Autodesk Inventor part; units mm, degrees
ref_plane "YZ Plane" through (0, 0, 0) normal (1, 0, 0) x (0, 1, 0)
ref_plane "XZ Plane" through (0, 0, 0) normal (0, 1, 0) x (-1, 0, 0)
ref_plane "XY Plane" through (0, 0, 0) normal (0, 0, 1) x (1, 0, 0)
sketch "Sketch2" plane through (0, 0, 0) normal (0, 0, 1) x (1, 0, 0)
  circle A0 centre (-22.5, 0) radius 1.2295
  circle A1 centre (11.25, -19.4856) radius 1.2295
  circle A2 centre (11.25, 19.4856) radius 1.2295
  circle A3 centre (22.5, 0) radius 1.2295
  circle A4 centre (-11.25, -19.4856) radius 1.2295
  circle A5 centre (-11.25, 19.4856) radius 1.2295
  circle A6 centre (0, 0) radius 25
  circle A7 centre (0, 0) radius 16
  circle A8 centre (0, 0) radius 15
  point P0 (0, 0)
extrude "Extrusion1" add sketch "Sketch2" along normal blind 2 contours A6 | A7
properties part number "P019-Joint_chambre_chapeau" material "Polytetrafluoroethylene"
Work out the finished part from the listing and answer in its coordinate system (mm). Give positions to 0.01 mm unless a question says otherwise; leave off trailing zeros. Loops run counter-clockwise (first coordinate to the right, second up) from the corner with the lowest first, then second, coordinate; pieces in that order, holes last. Notation, with made-up numbers: (62, 29.5) -> (107, 29.5) arc R21 cw to (107, 56.5) -> close; hole circle Ø3 at (15, 0). An arc over 180 degrees is marked (long way). Use a Markdown table: item, result. Add a question column.
1) For a pull along Y with two mould halves and no side action, classify faces 1 (the cylindrical face through (23.846, -7.509, 0.986)), 2 (the cylindrical face through (23.636, 0.471, 0.986)), 3 (the flat face through (11, -11, 0)) as +Y half, -Y half, draft (parallel to the pull), parting line (faces both ways), or undercut.
2) The part is cut by section D-D, the plane z = 1.55. Determine the outline of the cut face in (x, y), plus the area to 3 significant figures.
3) The part is cut by section B-B, the plane y = -3.5. Determine the outline of the cut face in (x, z), plus the area to 3 significant figures.
4) The part is cut by section C-C, the plane x = 11.25. Determine the outline of the cut face in (y, z), plus the area to 3 significant figures.
5) The part is cut by section A-A, the plane x = 0. Determine the outline of the cut face in (y, z).
6) Each of these flat-tipped pins is pushed along its axis until it touches: P1, Ø2, axis at x = 11.25, y = -19.49, coming from the +Z side; P2, Ø1, axis at y = -16, z = 0.5, coming from the -X side. Where does it stop, or does it pass through?
7) Consider line 1 along X through (y, z) = (19.5, 1.25); line 2 along Y through (x, z) = (-11.25, 0.75); line 3 along Y through (x, z) = (-8, 1.8). Determine where each line is inside the solid, lowest interval first.
Reported:
| question | item | result |
|---|---|---|
| 1 | face 1 | parting line |
| 1 | face 2 | undercut |
| 1 | face 3 | draft |
| 2 | outline | circle Ø50 at (0, 0); hole circle Ø2.46 at (-22.5, 0); hole circle Ø30 at (0, 0); hole circle Ø2.46 at (-11.25, -19.49); hole circle Ø2.46 at (-11.25, 19.49); hole circle Ø2.46 at (11.25, -19.49); hole circle Ø2.46 at (11.25, 19.49); hole circle Ø2.46 at (22.5, 0) |
| 2 | area | 1,230 mm^2 |
| 3 | outline | (-24.75, 0) -> (-14.59, 0) -> (-14.59, 2) -> (-24.75, 2) -> close; (14.59, 0) -> (24.75, 0) -> (24.75, 2) -> (14.59, 2) -> close |
| 3 | area | 40.7 mm^2 |
| 4 | outline | (-22.33, 0) -> (-20.72, 0) -> (-20.72, 2) -> (-22.33, 2) -> close; (-18.26, 0) -> (-9.92, 0) -> (-9.92, 2) -> (-18.26, 2) -> close; (9.92, 0) -> (18.26, 0) -> (18.26, 2) -> (9.92, 2) -> close; (20.72, 0) -> (22.33, 0) -> (22.33, 2) -> (20.72, 2) -> close |
| 4 | area | 39.8 mm^2 |
| 5 | outline | (-25, 0) -> (-15, 0) -> (-15, 2) -> (-25, 2) -> close; (15, 0) -> (25, 0) -> (25, 2) -> (15, 2) -> close |
| 6 | P1 | passes through |
| 6 | P2 | stops at x = -19.62 |
| 7 | line 1 | x = -15.64 to -12.48, -10.02 to 10.02, 12.48 to 15.64 |
| 7 | line 2 | y = -22.33 to -20.72, -18.26 to -9.92, 9.92 to 18.26, 20.72 to 22.33 |
| 7 | line 3 | y = -23.69 to -12.69, 12.69 to 23.69 |
